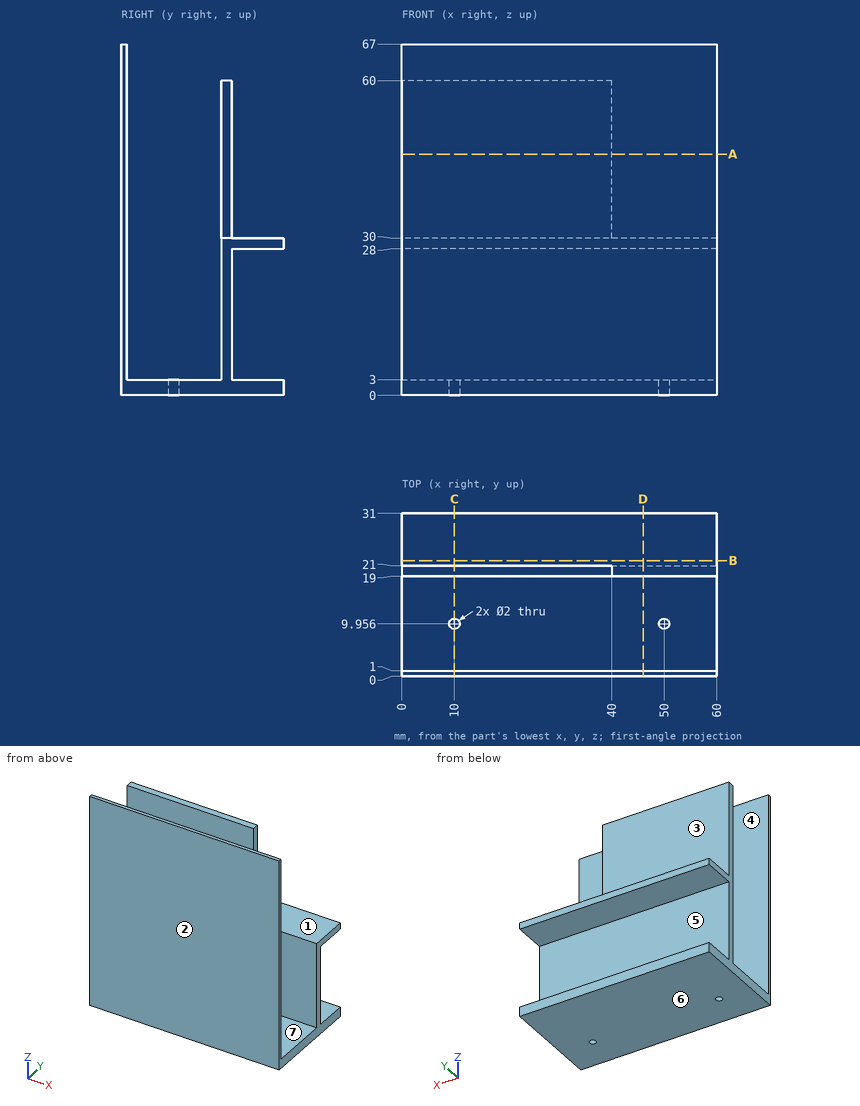
Answer from the drawing. Dimensions are ordinates in mm from the lowest x, y and z of the part. A direction names the side the tool comes from. Give positions to 0.01 mm unless a question says otherwise; leave off trailing zeros. Write each loop counter-clockwise with the first axis right and the second up, starting at its lowest first coordinate (ties: lowest second). Pieces come first, ordered by that corner, then holes. Notation, with made-up numbers: (-15.5, 37) - (7.5, 37) arc R17 ccw to (7.5, 50) - close; hole circle Ø7 at (57.25, -6). An arc over 180 degrees is marked (long way). Answer in a Markdown table with one row per item. Add a question column.
Item 1: Flat-ended cylindrical pins translate along their axes: P1, Ø1.5, axis at x = 29.5, y = 18, coming from the +Z side; P2, Ø12, axis at x = 28.5, z = 36, coming from the -Y side; P3, Ø12, axis at x = 34.5, z = 51, coming from the +Y side; P4, Ø5, axis at x = 47.5, y = 18, coming from the +Z side. Find the tip coordinate at first contact, or state that the pin passes through.
Item 2: A tool of negligible diameter and unlimited length cuts with its end or side. For the marked faces 5, 6 and 7, from which of +Z, -Z, +X, -X, +Y, -Y can it reach the whole face along a straight path? Write none if from no direction.
Item 3: Section D-D, the plane x = 46 is taken. Write down the section's boundary in (y, z), and give its area (3 significant figures).
Item 4: Section C-C, the plane x = 10 is taken. Write down the section's boundary in (y, z), and give its area (3 significant figures).
Item 5: Determine the mould class of the marked faces 1, 2, 3 and 4 for opening direction Y: pulls with the +Y half, pulls with the -Y half, needs draft (parallel to the pull), parting line crosses it, or undercut.
Item 6: Section A-A, the plane z = 46 is taken. Write down the section's boundary in (x, y), and give its area (3 significant figures).
Item 7: Find the intervals of material crossed by L1, parallel to Y at x = 18, z = 6; L2, parallel to Y at x = 10, z = 1; L3, parallel to Z at x = 17, y = 6.5, in increasing order.
Item 8: Section B-B, the plane y = 22 is taken. Write down the section's boundary in (x, z), and give its area (3 significant figures).
Recorded:
| question | item | result |
|---|---|---|
| 1 | P1 | stops at z = 3 |
| 1 | P2 | stops at y = 0 |
| 1 | P3 | stops at y = 21 |
| 1 | P4 | stops at z = 30 |
| 2 | face 5 | +X, -X, +Y |
| 2 | face 6 | -Z, +X, -X, +Y, -Y |
| 2 | face 7 | +Z, +X, -X |
| 3 | outline | (0, 0) - (31, 0) - (31, 3) - (21, 3) - (21, 28) - (31, 28) - (31, 30) - (19, 30) - (19, 3) - (1, 3) - (1, 67) - (0, 67) - close |
| 3 | area | 231 mm2 |
| 4 | outline | (0, 0) - (8.96, 0) - (8.96, 3) - (1, 3) - (1, 67) - (0, 67) - close; (10.96, 0) - (31, 0) - (31, 3) - (21, 3) - (21, 28) - (31, 28) - (31, 30) - (21, 30) - (21, 60) - (19, 60) - (19, 3) - (10.96, 3) - close |
| 4 | area | 285 mm2 |
| 5 | face 1 | needs draft |
| 5 | face 2 | pulls with the -Y half |
| 5 | face 3 | pulls with the +Y half |
| 5 | face 4 | undercut |
| 6 | outline | (0, 0) - (60, 0) - (60, 1) - (0, 1) - close; (0, 19) - (40, 19) - (40, 21) - (0, 21) - close |
| 6 | area | 140 mm2 |
| 7 | L1 | y = 0 to 1, 19 to 21 |
| 7 | L2 | y = 0 to 8.96, 10.96 to 31 |
| 7 | L3 | z = 0 to 3 |
| 8 | outline | (0, 0) - (60, 0) - (60, 3) - (0, 3) - close; (0, 28) - (60, 28) - (60, 30) - (0, 30) - close |
| 8 | area | 300 mm2 |
